```python
from build123d import *

# Parameters (mm, degrees)
F0_R     = 12.5
F0_R_2   = 7.5
F1_DEPTH = 25


with BuildPart() as f1:
    # F0 (on Top) → F1 (new body)
    with BuildSketch(Plane.XY):
        Polygon((0, -12.08159), (-70, -12.08159), (-70, -115), (32.5, -115), (57.5, -62.5), (57.5, 0), (80, 0), (80, 72.5), (-37.5, 72.5), (-37.5, 5.41841), (0, 5.41841), align=None)
        with Locations((-50, -100)):
            Circle(F0_R, mode=Mode.SUBTRACT)
        with Locations((-25, -75)):
            Circle(F0_R, mode=Mode.SUBTRACT)
        with Locations((0, -50)):
            Circle(F0_R, mode=Mode.SUBTRACT)
        with Locations((-22.5, 55)):
            Circle(F0_R_2, mode=Mode.SUBTRACT)
        with Locations((2.5, 55)):
            Circle(F0_R_2, mode=Mode.SUBTRACT)
        with Locations((22.5, 55)):
            Circle(F0_R_2, mode=Mode.SUBTRACT)
        with Locations((42.5, 55)):
            Circle(F0_R_2, mode=Mode.SUBTRACT)
        with Locations((62.5, 55)):
            Circle(F0_R_2, mode=Mode.SUBTRACT)
    extrude(amount=F1_DEPTH)


solid = f1.part
```
The model under review builds one solid part; all positions refer to its coordinate system, in mm. A direction names the side the tool comes from. Round coordinates to 2 decimals unless told otherwise and drop trailing zeros. Order: outer loops, then holes, each group sorted by start corner. A loop starts at its lowest first (then second) coordinate and runs counter-clockwise, first axis right, second up.
Item 1: For pin 1 (17 mm diameter, centred on x = 22.5, y = 55, fed in from -Z); pin 2 (10 mm diameter, centred on y = -37, z = 21.5, fed in from +X); pin 3 (14 mm diameter, centred on y = -2.5, z = 10, fed in from -X); pin 4 (11 mm diameter, centred on x = 74, z = 17, fed in from -Y), all flat-tipped, find the tip position at first contact; note any pin that passes through.
Working result:
pin 1: stops at z = 0
pin 2: stops at x = 57.5
pin 3: stops at x = 0
pin 4: stops at y = 0
Item 2: To check wall thickness, follow probe 1 along Y at (x, z) = (63, 14); probe 2 along Y at (x, z) = (-22.5, 9.5); probe 3 along X at (y, z) = (57.5, 14). State the ranges of each line that lie inside material, in increasing order.
Working result:
probe 1: y = 0 to 47.52, 62.48 to 72.5
probe 2: y = -115 to -87.25, -62.75 to -12.08, 5.42 to 47.5, 62.5 to 72.5
probe 3: x = -37.5 to -29.57, -15.43 to -4.57, 9.57 to 15.43, 29.57 to 35.43, 49.57 to 55.43, 69.57 to 80
Item 3: Draft analysis for pull direction Y (two halves, no side actions). For faces 1 (the cylindrical face through (55, 55, 12)), 2 (the flat face through (-19, -115, 12)), 3 (the flat face through (80, 36, 12)), state which applies: released by +Y, released by -Y, zero draft, split by the parting line, or undercut.
Working result:
face 1: undercut
face 2: released by -Y
face 3: zero draft
Item 4: Add section B-B, the plane y = 55. State the section outline as (x, z) points.
Working result:
outline: (-37.5, 0) - (-30, 0) - (-30, 25) - (-37.5, 25) - close; (-15, 0) - (-5, 0) - (-5, 25) - (-15, 25) - close; (10, 0) - (15, 0) - (15, 25) - (10, 25) - close; (30, 0) - (35, 0) - (35, 25) - (30, 25) - close; (50, 0) - (55, 0) - (55, 25) - (50, 25) - close; (70, 0) - (80, 0) - (80, 25) - (70, 25) - close
Item 5: Add section C-C, the plane z = 19.75. Count the separate pieces of the cut face and the enclosed holes in it, and give its area (3 significant figures).
Working result:
separate pieces: 1
enclosed holes: 8
area: 19,100 mm2
Item 6: Machinability: for faces 4 (the flat face through (-37.5, 39, 12)), 5 (the cylindrical face through (-51.627, -87.606, 12.325)), 6 (the flat face through (0, -3, 12)), 7 (the flat face through (57.5, -32, 12)), which of the approach directions +Z, -Z, +X, -X, +Y, -Y give a long, thin tool a straight path to every point of the face, cutting with its end or side? Answer none if there is none.
Working result:
face 4: +Z, -Z, -X, +Y
face 5: +Z, -Z
face 6: +Z, -Z, -X
face 7: +Z, -Z, +X, -Y
Item 7: Add section D-D, the plane x = -26. State the section outline as (y, z) points.
Working result:
outline: (-115, 0) - (-87.46, 0) - (-87.46, 25) - (-115, 25) - close; (-62.54, 0) - (-12.08, 0) - (-12.08, 25) - (-62.54, 25) - close; (5.42, 0) - (48.37, 0) - (48.37, 25) - (5.42, 25) - close; (61.63, 0) - (72.5, 0) - (72.5, 25) - (61.63, 25) - close
Item 8: Add section A-A, the plane x = 42.5. State the section outline as (y, z) points, and give its area (3 significant figures).
Working result:
outline: (-94, 0) - (47.5, 0) - (47.5, 25) - (-94, 25) - close; (62.5, 0) - (72.5, 0) - (72.5, 25) - (62.5, 25) - close
area: 3,790 mm2
